Here's how the part is built. I have some questions about the finished solid (model axes, mm). A direction names the side the tool comes from. Round coordinates to 2 decimals unless told otherwise and drop trailing zeros. Order: outer loops, then holes, each group sorted by start corner. A loop starts at its lowest first (then second) coordinate and runs counter-clockwise, first axis right, second up.
```python
from build123d import *

# Parameters (mm, degrees)
BOSS_EXTRU_1_DEPTH      = 6
ESQUISSE2_R             = 4.1
ENL_V_MAT_EXTRU_1_DEPTH = 1.22
ENL_V_MAT_EXTRU_2_REACH = 191.832
ESQUISSE3_R             = 3.1
ENL_V_MAT_EXTRU_3_REACH = 191.832
ESQUISSE5_W             = 9.4
ESQUISSE5_H             = 3.5
CONG_1_R                = 1


with BuildPart() as part:
    # Esquisse1 → Boss.-Extru.1 (new body)
    with BuildSketch(Plane.XY):
        with BuildLine():
            Line((120, -60), (-120, -60))
            ThreePointArc((-120, -60), (-180, 0), (-120, 60))
            Line((-120, 60), (120, 60))
            ThreePointArc((120, 60), (180, 0), (120, -60))
        make_face()
    extrude(amount=BOSS_EXTRU_1_DEPTH)

    # Esquisse2 → Enlèv. mat.-Extru.1 (cut)
    with BuildSketch(Plane.XY.offset(6)):
        with Locations((-35.893989476, 43.512538926)):
            Circle(ESQUISSE2_R)
        with Locations((35.893989476, 43.512538926)):
            Circle(ESQUISSE2_R)
        with Locations((35.893989476, -43.512538926)):
            Circle(ESQUISSE2_R)
        with Locations((-35.893989476, -43.512538926)):
            Circle(ESQUISSE2_R)
    extrude(amount=-ENL_V_MAT_EXTRU_1_DEPTH, mode=Mode.SUBTRACT)

    # Esquisse3 → Enlèv. mat.-Extru.2 (cut, up to next)
    with BuildSketch(Plane(origin=(0, 0, 0), x_dir=(-1, 0, 0), z_dir=(0, 0, -1)), mode=Mode.PRIVATE) as enl_v_mat_extru_2_sk1:
        with Locations((12.25, -34.19)):
            Circle(ESQUISSE3_R)
    enl_v_mat_extru_2_tool1 = extrude(enl_v_mat_extru_2_sk1.sketch, amount=-ENL_V_MAT_EXTRU_2_REACH, mode=Mode.PRIVATE) & part.part
    add(enl_v_mat_extru_2_tool1.solids().sort_by_distance((-12.25, -34.19, 0))[0], mode=Mode.SUBTRACT)

    # Esquisse5 → Enlèv. mat.-Extru.3 (cut, up to next)
    with BuildSketch(Plane.XY.offset(6), mode=Mode.PRIVATE) as enl_v_mat_extru_3_sk1:
        with Locations((-12.25, -45.54)):
            Rectangle(ESQUISSE5_W, ESQUISSE5_H)
    enl_v_mat_extru_3_tool1 = extrude(enl_v_mat_extru_3_sk1.sketch, amount=-ENL_V_MAT_EXTRU_3_REACH, mode=Mode.PRIVATE) & part.part
    add(enl_v_mat_extru_3_tool1.solids().sort_by_distance((-12.25, -45.54, 6))[0], mode=Mode.SUBTRACT)

    # Congé1
    cong_1_edges = [part.edges().sort_by_distance(p)[0] for p in [
        (-7.55, -43.79, 3),
        (-7.55, -47.29, 3),
        (-16.95, -47.29, 3),
        (-16.95, -43.79, 3),
    ]]
    fillet(cong_1_edges, radius=CONG_1_R)


solid = part.part
```
1. I'm going to push flat-ended pins straight in: P1, Ø9.5, axis at x = -35.89, y = -43.51, coming from the +Z side; P2, Ø5, axis at x = -35.89, y = 43.51, coming from the +Z side; P3, Ø0.8, axis at y = -46, z = 2, coming from the -X side; P4, Ø5, axis at x = -12.25, y = -34.19, coming from the -Z side. Where does each tip first touch, or does it pass through?
Evaluation:
P1: stops at z = 6
P2: stops at z = 4.78
P3: stops at x = -159
P4: passes through
2. If we section it at B-B, the plane y = -34.19: Write out the boundary of the cut face in (x, z).
Evaluation:
outline: (-169.31, 0) - (-15.35, 0) - (-15.35, 6) - (-169.31, 6) - close; (-9.15, 0) - (169.31, 0) - (169.31, 6) - (-9.15, 6) - close
3. If we section it at A-A, the plane x = -12.25: Write out the boundary of the cut face in (y, z), and give its area (3 significant figures).
Evaluation:
outline: (-60, 0) - (-47.29, 0) - (-47.29, 6) - (-60, 6) - close; (-43.79, 0) - (-37.29, 0) - (-37.29, 6) - (-43.79, 6) - close; (-31.09, 0) - (60, 0) - (60, 6) - (-31.09, 6) - close
area: 662 mm2
4. On a 3-axis mill with a long thin cutter (end or side, diameter ignored), from which of +Z, -Z, +X, -X, +Y, -Y can I reach the whole of each face in a straight line? I mean faces 5 (the flat face through (-12, -43.79, 3)), 6 (the flat face through (36, 44, 4.78)), 7 (the cylindrical face through (179.985, 1.319, 2.958)). Say none if no direction works.
Evaluation:
face 5: +Z, -Z
face 6: +Z
face 7: +Z, -Z, +X
5. I need wall thicknesses on probe 1 along Y at (x, z) = (-12.5, 2.05); probe 2 along X at (y, z) = (-32, 0.55); probe 3 along X at (y, z) = (26, 3.2). Which ranges of each line are inside material? Lowest first, please.
Evaluation:
probe 1: y = -60 to -47.29, -43.79 to -37.28, -31.1 to 60
probe 2: x = -170.75 to -14.44, -10.06 to 170.75
probe 3: x = -174.07 to 174.07
6. If we section it at C-C, the plane z = 3.75: Write out the boundary of the cut face in (x, y), and give its area (3 significant figures).
Evaluation:
outline: (-120, -60) - (120, -60) arc R60 ccw to (120, 60) - (-120, 60) arc R60 ccw to start; hole (-16.95, -46.29) arc R1 ccw to (-15.95, -47.29) - (-8.55, -47.29) arc R1 ccw to (-7.55, -46.29) - (-7.55, -44.79) arc R1 ccw to (-8.55, -43.79) - (-15.95, -43.79) arc R1 ccw to (-16.95, -44.79) - close; hole circle Ø6.2 at (-12.25, -34.19)
area: 40,000 mm2
7. If we mould it in two halves opening along Y, with no side actions, what happens to faces 1 (the cylindrical face through (-179.985, -1.319, 2.958)), 2 (the cylindrical face through (-39.99, 43.69, 5.4)), 3 (the flat face through (3, 1, 6)), 4 (the flat face through (2, -60, 3))? For each: released by +Y, released by -Y, zero draft, split by the parting line, or undercut.
Evaluation:
face 1: split by the parting line
face 2: undercut
face 3: zero draft
face 4: released by -Y
